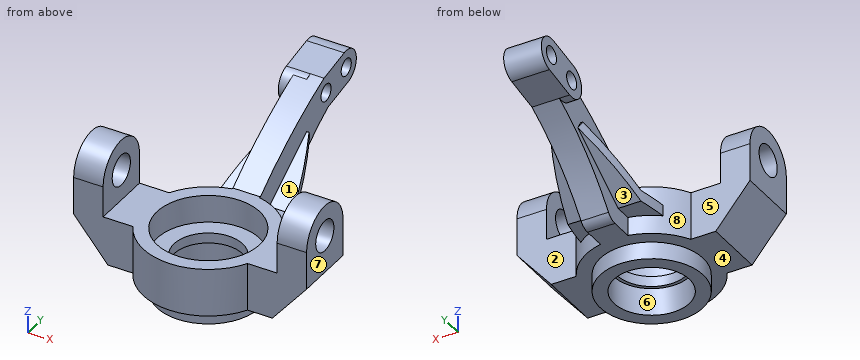
Autodesk Inventor part; units mm, degrees
ref_plane "YZ Plane" through (0, 0, 0) normal (1, 0, 0) x (0, 1, 0)
ref_plane "XZ Plane" through (0, 0, 0) normal (0, 1, 0) x (-1, 0, 0)
ref_plane "XY Plane" through (0, 0, 0) normal (0, 0, 1) x (1, 0, 0)
sketch "Sketch1" plane through (0, 0, 0) normal (0, 0, 1) x (1, 0, 0)
  line L0 (17, 4.5) -> (17, -4.5)
  line L1 (-17, -4.5) -> (-17, 4.5)
  arc A0 (-8.3666, -4.5) -> (8.3666, -4.5) centre (0, 0) ccw
  arc A1 (8.3666, 4.5) -> (-8.3666, 4.5) centre (0, 0) ccw
  line L2 (-17, 4.5) -> (-8.3666, 4.5)
  line L3 (8.3666, 4.5) -> (17, 4.5)
  line L4 (17, -4.5) -> (8.3666, -4.5)
  line L5 (-8.3666, -4.5) -> (-17, -4.5)
  line L6 (-17, 4.5) -> (17, -4.5) construction
  line L7 (-17, -4.5) -> (17, 4.5) construction
  point P0 (0, 0)
  point P1 (0, 0)
  dimension "d0" = 9
  dimension "d1" = 34
  dimension "d2" = 9.5
  dimension "d3" = 9
  dimension "d4" = 9.5
  dimension "d12" = 4.5
extrude "Extrusion1" add sketch "Sketch1" along normal blind 7
sketch "Sketch2" plane through (17, -4.5, 0) normal (1, 0, 0) x (0, 0, -1)
  arc A0 (-11.5, 9) -> (-11.5, 0) centre (-11.5, 4.5) ccw
  circle A1 centre (-11.5, 4.5) radius 2.25
  line L0 (-7, 9) -> (-11.5, 9)
  line L1 (-11.5, 0) -> (-7, 0)
  line L2 (-7, 0) -> (-7, 9)
  point P0 (0, 4.5)
  point P1 (-7, 0)
  dimension "d7" = 9
  dimension "d8" = 4.5
  dimension "d9" = 9
extrude "Extrusion2" add sketch "Sketch2" against normal blind 4.3
extrude "Extrusion3" add sketch "Sketch2" along normal blind 4.3 from surface at -34
sketch "Sketch3" plane through (-17, -4.5, 0) normal (0, -1, 0) x (1, 0, 0)
  line L0 (0, 6) -> (0, 0)
  line L1 (0, 0) -> (5, 0)
  line L2 (5, 0) -> (0, 6)
  line L3 (29, 0) -> (34, 0)
  line L4 (34, 0) -> (34, 6)
  line L5 (34, 6) -> (29, 0)
  point P0 (17, 0)
  dimension "d15" = 6
  dimension "d16" = 5
  dimension "d17" = 6
  dimension "d18" = 5
extrude "Extrusion4" cut sketch "Sketch3" against normal up to next
sketch "Sketch4" plane through (0, 0, 0) normal (0, 0, -1) x (-1, 0, 0)
  circle A0 centre (0, 0) radius 7.5
  dimension "d21" = 15
extrude "Extrusion5" add sketch "Sketch4" along normal blind 2.5
sketch "Sketch5" plane through (0, 0, 7) normal (0, 0, 1) x (1, 0, 0)
  circle A0 centre (0, 0) radius 7.5
  dimension "d24" = 15
extrude "Extrusion6" cut sketch "Sketch5" against normal blind 4
sketch "Sketch6" plane through (0, 0, -2.5) normal (0, 0, -1) x (-1, 0, 0)
  circle A0 centre (0, 0) radius 5.5
  dimension "d27" = 11
extrude "Extrusion7" cut sketch "Sketch6" against normal blind 4
sketch "Sketch7" plane through (0, 0, 1.5) normal (0, 0, -1) x (-1, 0, 0)
  circle A0 centre (0, 0) radius 5
  dimension "d30" = 10
extrude "Extrusion8" cut sketch "Sketch7" against normal up to next
sketch "Sketch9" plane through (0, 0, 0) normal (1, 0, 0) x (0, 1, 0)
  line L0 (-9.5504, 0) -> (57.3026, 0)
  line L1 (0, -37.6235) -> (0, 29.8791)
  line L2 (9.5, 0) -> (4.5, 0)
  line L3 (9.5, 7) -> (4.5, 7)
  circle A0 centre (30.75, 14.5) radius 1.25
  circle A1 centre (25.75, 13.5) radius 1.25
  line L4 (8.5, 7) -> (9.5, 7)
  line L5 (13.5, 7) -> (13.5, 0) construction
  line L6 (12.4966, 0) -> (8.5, 0)
  line L7 (8.5, 0) -> (8.5, 7)
  line L8 (25.75, 13.5) -> (30.75, 14.5) construction
  line L9 (26.2403, 11.0485) -> (31.2403, 12.0485)
  line L10 (30.2597, 16.9515) -> (25.2597, 15.9515)
  arc A2 (25.2597, 15.9515) -> (26.2403, 11.0485) centre (25.75, 13.5) ccw construction
  arc A3 (31.2403, 12.0485) -> (30.2597, 16.9515) centre (30.75, 14.5) ccw
  arc A4 (25.2597, 15.9515) -> (9.5, 7) centre (49.2826, -44.6916) ccw
  arc A5 (26.2403, 11.0485) -> (14.0842, 0.7836) centre (43.5805, -21.8166) ccw
  arc A6 (12.4966, 0) -> (14.0842, 0.7836) centre (12.4966, 2) ccw
  point P0 (0, 0)
  point P1 (28.25, 14)
  dimension "d133" = 2.5
  dimension "d134" = 30.75
  dimension "d135" = 14.5
  dimension "d136" = 2.5
  dimension "d137" = 13.5
  dimension "d138" = 25.75
  dimension "d139" = 7
  dimension "d140" = 5
  dimension "d141" = 8.5
  dimension "d142" = 5
  dimension "d143" = 65.2279
  dimension "d144" = 37.1592
  dimension "d145" = 2
extrude "Extrusion22" add sketch "Sketch9" along normal mid plane 4
sketch "Sketch19" plane through (0, 0, 0) normal (1, 0, 0) x (0, 1, 0)
  circle A0 centre (25.75, 13.5) radius 1.25
  circle A1 centre (25.75, 13.5) radius 1.25
  circle A2 centre (30.75, 14.5) radius 1.25
  circle A3 centre (30.75, 14.5) radius 1.25
  line L0 (25.75, 13.5) -> (30.75, 14.5) construction
  line L1 (26.2403, 11.0485) -> (31.2403, 12.0485)
  line L2 (30.2597, 16.9515) -> (25.2597, 15.9515)
  arc A4 (25.2597, 15.9515) -> (26.2403, 11.0485) centre (25.75, 13.5) ccw
  arc A5 (31.2403, 12.0485) -> (30.2597, 16.9515) centre (30.75, 14.5) ccw
  point P0 (0, 0)
  point P1 (28.25, 14)
  dimension "d148" = 2.5
  dimension "d149" = 2.5
  dimension "d150" = 5
extrude "Extrusion23" add sketch "Sketch19" against normal blind 3.5
sketch "Sketch20" plane through (0, 0, 0) normal (1, 0, 0) x (0, 1, 0)
  line L0 (0, 4.3) -> (11.7, 4.3)
  line L1 (11.7, 4.3) -> (11.7, 2.7) construction
  line L2 (11.7, 2.7) -> (0, 2.7)
  line L3 (0, 2.7) -> (0, 4.3)
  line L4 (-18.05, 0) -> (41.8, 0)
  line L5 (0, -6.4) -> (0, 20.9)
  line L6 (11.7, 2.7) -> (21.7, 9.2)
  line L7 (11.7, 4.3) -> (20.9843, 10.3348)
  line L8 (20.9843, 10.3348) -> (21.7, 9.2)
  point P0 (0, 0)
  dimension "d153" = 1.6
  dimension "d154" = 11.7
  dimension "d155" = 2.7
  dimension "d156" = 10
  dimension "d157" = 6.5
  dimension "d158" = 1.1348
extrude "Extrusion24" add sketch "Sketch20" along normal mid plane 12
sketch "Sketch21" plane through (0, 0, 7) normal (0, 0, 1) x (1, 0, 0)
  circle A0 centre (0, 0) radius 7.5
  dimension "d161" = 15
extrude "Extrusion25" cut sketch "Sketch5" against normal blind 4
sketch "Sketch22" plane through (0, 0, 1.5) normal (0, 0, -1) x (-1, 0, 0)
  circle A0 centre (0, 0) radius 5
  dimension "d164" = 10
extrude "Extrusion26" cut sketch "Sketch22" against normal through all
sketch "Sketch23" plane through (0, 0, 0) normal (0, 0, 1) x (1, 0, 0)
  line L0 (-6, 21.7) -> (-2, 21.7)
  line L1 (-6, 21.7) -> (-6, 11.7)
  line L2 (-2, 21.7) -> (-6, 21.7)
  line L3 (-6, 7.3655) -> (-6, 11.7)
  line L4 (-6, 21.7) -> (-6, 7.3655)
  arc A0 (-2, 21.7) -> (-6, 7.3655) centre (37.8943, 2.8423) ccw
  line L5 (0, 17.7237) -> (0, 15.5632) construction
  line L6 (6, 21.7) -> (2, 21.7)
  line L7 (6, 21.7) -> (6, 11.7)
  line L8 (6, 7.3655) -> (6, 11.7)
  arc A1 (6, 7.3655) -> (2, 21.7) centre (-37.8943, 2.8423) ccw
  point P0 (0, 0)
extrude "Extrusion27" cut sketch "Sketch23" along normal through all
properties part number "RCT-P006_steering_knuckle"
Design review of the part built by this model. Coordinates are the model's own, in mm. Face numbers are marked on the shaded views. A direction names the side the tool comes from. Coordinates: 2 decimals unless noted, no trailing zeros. Write each loop counter-clockwise with the first axis right and the second up, starting at its lowest first coordinate (ties: lowest second). Pieces come first, ordered by that corner, then holes. Notation, with made-up numbers: M 71.25,47.25 L 120.25,47.25 A16 cw 120.25,76.25 Z; hole C -18,39 d3. An arc over 180 degrees is marked long. Answer as a JSON object with one key per item and string values.
Item 1: Add section A-A, the plane y = 0. State how many separate pieces and enclosed holes the cut face has, and give its area (3 significant figures).
Outcome:
{"separate pieces": "4", "enclosed holes": "0", "area": "165 mm²"}
Item 2: Add section B-B, the plane x = 4.5. Give the boundary of the cut face in (y, z).
Outcome:
{"outline": "M -8.37,0 L -6,0 L -6,-2.5 L -3.16,-2.5 L -3.16,1.5 L -2.18,1.5 L -2.18,3 L -6,3 L -6,7 L -8.37,7 Z; M 2.18,1.5 L 3.16,1.5 L 3.16,-2.5 L 6,-2.5 L 6,0 L 8.37,0 L 8.37,2.7 L 11.7,2.7 L 15.09,4.9 L 15.09,6.5 L 11.7,4.3 L 8.37,4.3 L 8.37,7 L 6,7 L 6,3 L 2.18,3 Z"}
Item 3: Wall thickness on probe 1 along Y at (x, z) = (0, -1.2); probe 2 along X at (y, z) = (24, 11.75); probe 3 along Y at (x, z) = (1, 0.5): over which ranges is each line inside the solid? List them lowest first.
Outcome:
{"probe 1": "-7.5 to -5.5, 5.5 to 7.5", "probe 2": "-3.5 to 2", "probe 3": "-9.45 to -5.41, 5.41 to 13.82"}
Item 4: Machinability: for the marked faces 1, 2, 3 and 4, which of the approach directions +Z, -Z, +X, -X, +Y, -Y give a long, thin tool a straight path to every point of the face, cutting with its end or side? Answer none if there is none.
Outcome:
{"face 1": "+Z, +X", "face 2": "+Z, -Z, +X, +Y", "face 3": "-Z, -X, +Y", "face 4": "-Z"}
Item 5: Draft analysis for pull direction Y (two halves, no side actions). For the marked faces 5, 6, 7 and 8, state which applies: pulls with the +Y half, pulls with the -Y half, needs draft (parallel to the pull), parting line crosses it, or undercut.
Outcome:
{"face 5": "pulls with the +Y half", "face 6": "undercut", "face 7": "needs draft", "face 8": "undercut"}
Item 6: Insertion check: pin 1 Ø3 at (y, z) = (30.75, 14.5) entering from +X; pin 2 Ø6 at (x, z) = (13, 1.5) entering from +Y; pin 3 Ø9.5 at (x, z) = (12.5, 5) entering from -Y. Each pin has a flat end and moves straight along its axis. Give the tip position at first contact, or say it passes through.
Outcome:
{"pin 1": "x = 2", "pin 2": "y = 4.5", "pin 3": "y = -5.49"}
Item 7: Add section C-C, the plane x = -13.5. Give the boundary of the cut face in (y, z), and give its area (3 significant figures).
Outcome:
{"outline": "M -4.5,1.8 L 4.5,1.8 L 4.5,11.5 A4.5 ccw -4.5,11.5 Z; hole C 0,11.5 d4.5", "area": "103 mm²"}
Item 8: Add section D-D, the plane y = 30.75. Give the boundary of the cut face in (x, z).
Outcome:
{"outline": "M -3.5,11.95 L 2,11.95 L 2,13.25 L -3.5,13.25 Z; M -3.5,15.75 L 2,15.75 L 2,17 L -3.5,17 Z"}
